Input: part model. Units: mm. Frame: model coordinates. Face numbers are marked on the shaded views. A direction names the side the tool comes from. Round coordinates to 2 decimals unless told otherwise and drop trailing zeros. Order: outer loops, then holes, each group sorted by start corner. A loop starts at its lowest first (then second) coordinate and runs counter-clockwise, first axis right, second up. Notation, with made-up numbers: (20, 28.25) - (24, 28.25) arc R19 ccw to (24, 39.25) - close; hole circle Ø10 at (-5, 30.5). An arc over 180 degrees is marked (long way). One line per item, written item: value. Start each with the question number.
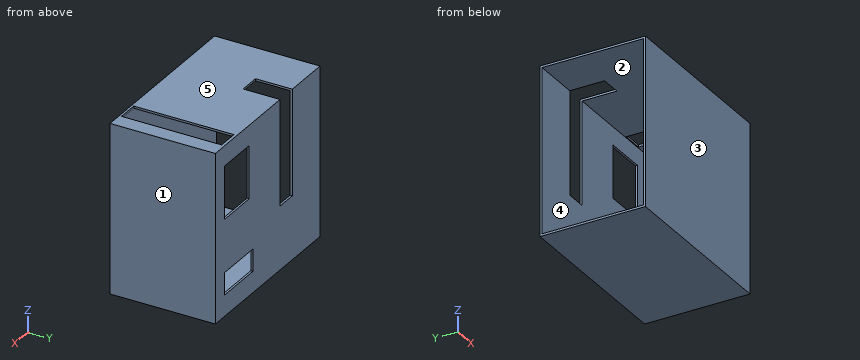
from build123d import *

# Parameters (mm, degrees)
SKETCH1_W           = 200
SKETCH1_H           = 100
BOSS_EXTRUDE1_DEPTH = 160
SHELL3_T            = -2
SKETCH2_W           = 46
SKETCH2_H           = 21
SKETCH2_W_2         = 40
SKETCH2_H_2         = 50
CUT_EXTRUDE1_DEPTH  = 68
SKETCH4_W           = 20
SKETCH4_H           = 95
CUT_EXTRUDE2_DEPTH  = 18
SKETCH6_W           = 20
SKETCH6_H           = 100
CUT_EXTRUDE3_DEPTH  = 35
SKETCH8_W           = 167.837082792
SKETCH8_H           = 105.374637329
CUT_EXTRUDE4_DEPTH  = 30


with BuildPart() as part:
    # Sketch1 → Boss-Extrude1 (new body)
    with BuildSketch(Plane.XY):
        with Locations((32.679929783, -17.656524283)):
            Rectangle(SKETCH1_W, SKETCH1_H)
    extrude(amount=BOSS_EXTRUDE1_DEPTH)

    # Shell3
    shell3_openings = [part.faces().sort_by_distance(p)[0] for p in [
        (-67.320070217, -17.656524283, 80),
    ]]
    offset(amount=SHELL3_T, openings=shell3_openings, kind=Kind.INTERSECTION)

    # Sketch2 → Cut-Extrude1 (cut)
    with BuildSketch(Plane(origin=(0, 32.343475717, 0), x_dir=(1, 0, 0), z_dir=(0, 1, 0))):
        with Locations((94.679929783, -30.5)):
            Rectangle(SKETCH2_W, SKETCH2_H)
        with Locations((97.679929783, -116)):
            Rectangle(SKETCH2_W_2, SKETCH2_H_2)
    extrude(amount=-CUT_EXTRUDE1_DEPTH, mode=Mode.SUBTRACT)

    # Sketch4 → Cut-Extrude2 (cut)
    with BuildSketch(Plane.XY.offset(160)):
        with Locations((107.679929783, -18.012169352)):
            Rectangle(SKETCH4_W, SKETCH4_H)
    extrude(amount=-CUT_EXTRUDE2_DEPTH, mode=Mode.SUBTRACT)

    # Sketch6 → Cut-Extrude3 (cut)
    with BuildSketch(Plane(origin=(0, 32.343475717, 0), x_dir=(1, 0, 0), z_dir=(0, 1, 0))):
        with Locations((17.679929783, -110)):
            Rectangle(SKETCH6_W, SKETCH6_H)
    extrude(amount=-CUT_EXTRUDE3_DEPTH, mode=Mode.SUBTRACT)

    # Sketch8 → Cut-Extrude4 (cut)
    with BuildSketch(Plane.ZY.offset(67.320070217)):
        with Locations((79.323733366, -18.148354562)):
            Rectangle(SKETCH8_W, SKETCH8_H)
    extrude(amount=-CUT_EXTRUDE4_DEPTH, mode=Mode.SUBTRACT)


solid = part.part
Item 1: Section query A-A on y = 0.5. Return loops of the section in (x, z), and give its area (3 significant figures).
Item 2: First-contact query: pin 1 Ø2 at (x, z) = (13, 159.5) entering from +Y; pin 2 Ø1 at (y, z) = (-52, 74.5) entering from -X; pin 3 Ø2 at (x, y) = (20, 31.5) entering from +Z. Flat tips, straight axial feed; report the tip coordinate or a pass-through.
Item 3: Line query: L1, parallel to Z at x = 81, y = -10; L2, parallel to Y at x = 28, z = 22; L3, parallel to X at y = -32, z = 30. Output: solid intervals per line, ascending.
Item 4: Section query B-B on z = 137.5. Return loops of the section in (x, y).
Item 5: Pull-direction query (Y, two-part tool) for the marked faces 3, 4 and 5; classes: released by +Y, released by -Y, zero draft, split by the parting line, or undercut.
Item 6: Section query C-C on x = 11. Return loops of the section in (y, z), and give its area (3 significant figures).
Item 7: Reachability of the marked faces 1 and 2 from +Z, -Z, +X, -X, +Y, -Y: full face, straight path, thin tool, end or side. Return the list, or none.
Item 8: Section query D-D on z = 72.5. Return loops of the section in (x, y), and give its area (3 significant figures).
Geometry results:
1. outline: (-37.32, 0) - (132.68, 0) - (132.68, 160) - (117.68, 160) - (117.68, 158) - (130.68, 158) - (130.68, 2) - (-37.32, 2) - close; (-37.32, 158) - (7.68, 158) - (7.68, 160) - (-37.32, 160) - close; (27.68, 158) - (97.68, 158) - (97.68, 160) - (27.68, 160) - close
1. area: 912 mm^2
2. pin 1: stops at y = -2.66
2. pin 2: stops at x = 130.68
2. pin 3: stops at z = 60
3. L1: z = 0 to 2, 158 to 160
3. L2: y = -67.66 to -65.66, 30.34 to 32.34
3. L3: x = 130.68 to 132.68
4. outline: (-37.32, -67.66) - (132.68, -67.66) - (132.68, 32.34) - (117.68, 32.34) - (117.68, 30.34) - (130.68, 30.34) - (130.68, -65.66) - (-37.32, -65.66) - close; (-37.32, 30.34) - (7.68, 30.34) - (7.68, 32.34) - (-37.32, 32.34) - close; (27.68, 30.34) - (77.68, 30.34) - (77.68, 32.34) - (27.68, 32.34) - close
5. face 3: released by -Y
5. face 4: undercut
5. face 5: zero draft
6. outline: (-67.66, 0) - (32.34, 0) - (32.34, 60) - (30.34, 60) - (30.34, 2) - (-65.66, 2) - (-65.66, 158) - (-2.66, 158) - (-2.66, 160) - (-67.66, 160) - close
6. area: 758 mm^2
7. face 1: +Z, -Z, +X, +Y, -Y
7. face 2: -X
8. outline: (-37.32, -67.66) - (132.68, -67.66) - (132.68, 32.34) - (27.68, 32.34) - (27.68, 30.34) - (130.68, 30.34) - (130.68, -65.66) - (-37.32, -65.66) - close; (-37.32, 30.34) - (7.68, 30.34) - (7.68, 32.34) - (-37.32, 32.34) - close
8. area: 832 mm^2
